Autodesk Inventor part; units mm, degrees
ref_plane "Work Plane2" through (-20, -2, 5) normal (0, 0, 1) x (1, 0, 0)
ref_plane "YZ Plane" through (0, 0, 0) normal (1, 0, 0) x (0, 1, 0)
ref_plane "XZ Plane" through (0, 0, 0) normal (0, 1, 0) x (-1, 0, 0)
sketch "Sketch1" plane through (0, 0, 0) normal (0, 1, 0) x (-1, 0, 0)
  line L0 (0, 0) -> (30, 0)
  line L1 (0, 5) -> (0, 0)
  line L2 (20, 5) -> (30, 0)
  line L3 (30, 12) -> (0, 12)
  line L4 (0, 12) -> (0, 5)
  line L5 (0, 5) -> (0, 7)
  line L6 (18, 7) -> (30, 12)
  line L7 (20, 5) -> (10, 5)
  line L8 (10, 5) -> (10, 7)
  line L9 (18, 7) -> (10, 7)
  line L10 (10, 5) -> (0, 5)
  line L11 (10, 5) -> (10, 0)
  dimension "d13" = 2
  dimension "d15" = 10
extrude "Extrusion2" add sketch "Sketch1" along normal blind 30 contours L1 L10 L11 L0 | L11 L7 L2 L0
ref_plane "Work Plane2" through (-20, -2, 5) normal (0, 0, 1) x (1, 0, 0)
sketch "Sketch2" plane through (-20, -2, 5) normal (0, 0, 1) x (1, 0, 0)
  line L0 (20, 2) -> (20, 17)
  line L1 (20, 2) -> (20, 32)
  line L2 (20, 17) -> (10, 17)
  circle A0 centre (10, 17) radius 5
  circle A1 centre (10, 17) radius 7.5
  line L3 (20, 32) -> (15, 32)
  line L4 (20, 32) -> (-10, 32)
  line L5 (15, 32) -> (15, 27)
  circle A2 centre (15, 27) radius 2.25
  line L6 (20, 17) -> (20, 7)
  line L7 (20, 2) -> (20, 32)
  line L8 (20, 7) -> (15, 7)
  circle A3 centre (15, 7) radius 2.25
  dimension "d20" = 10
  dimension "d21" = 10
  dimension "d22" = 15
  dimension "d30" = 5
  dimension "d31" = 5
  dimension "d32" = 4.5
  dimension "d33" = 10
  dimension "d34" = 5
  dimension "d35" = 4.5
extrude "Extrusion3" cut sketch "Sketch2" against normal blind 3 contours A0
fillet "Fillet3" radius 3 2 edges at (-15, 15, 5) (-15, 15, 2)
extrude "Extrusion4" add sketch "Sketch1" against normal blind 2 contours L11 L7 L2 L0
extrude "Extrusion5" cut sketch "Sketch2" against normal blind 20 contours A2 | A3
properties part number "clip_tip"
For this review, take the finished solid that the model builds, in its own axes (mm). A direction names the side the tool comes from. Coordinates: 2 decimals unless noted, no trailing zeros. Write each loop counter-clockwise with the first axis right and the second up, starting at its lowest first coordinate (ties: lowest second). Pieces come first, ordered by that corner, then holes. Notation, with made-up numbers: (84.5, 53.5) -> (136.5, 53.5) arc R15 cw to (136.5, 81.5) -> close; hole circle Ø5 at (-32.5, 78.5). An arc over 180 degrees is marked (long way). Write each question's results on one line, items separated by ' | '. Start each with the question number.
1) Consider section D-D (z = 4.5). Write out the cut boundary in (x, y), plus the area to 3 significant figures.
2) Consider section A-A (z = 0.9). Write out the cut boundary in (x, y).
3) Consider section C-C (x = -6). Give the number of separate pieces and of enclosed holes in the cut face, plus the area to 3 significant figures.
4) Insertion check: pin 1 (1.5 mm diameter, centred on x = -5, y = 16, fed in from +Z); pin 2 (7 mm diameter, centred on x = -5, y = 5, fed in from -Z); pin 3 (3 mm diameter, centred on x = -6.5, z = 4.5, fed in from -Y); pin 4 (1.5 mm diameter, centred on x = -22, y = 7, fed in from +Z) (3 decimals). Each pin has a flat end and moves straight along its axis. Give the tip position at first contact, or say it passes through.
5) For faces 1 (the face through (-18, -2, 3)), 2 (the face through (-10, -1, 3)), 3 (the face through (-10, 15, 2)), list the 3-axis set-ups (+Z, -Z, +X, -X, +Y, -Y) from which the entire face can be reached by the end or side of a thin tool; tool diameter is ignored.
6) Consider section B-B (y = 25). Write out the cut boundary in (x, z), plus the area to 4 significant figures.
7) Wall thickness on L1, parallel to Y at x = -5, z = 1.45; L2, parallel to Y at x = -3, z = 2.65; L3, parallel to Y at x = -6, z = 4.5: over which ranges is each line inside the solid? List them lowest first. Write a range as [from, to].
8) The part is to be moulded in two halves that separate along X. For faces 4 (the face through (-2.854, 5.676, 2.535)), 5 (the face through (-11, 30, 3)), 6 (the face through (-5.488, 22.804, 2.535)), 7 (the face through (-24.93, 14.224, 2.535)), say which applies: +X half, -X half, draft (parallel to the pull), parting line (faces both ways), or undercut.
Geometry says:
1) outline: (-21, -2) -> (-10, -2) -> (-10, 0) -> (0, 0) -> (0, 30) -> (-21, 30) -> close; hole circle Ø12.68 at (-10, 15); hole circle Ø4.5 at (-5, 5); hole circle Ø4.5 at (-5, 25) | area: 494 mm^2
2) outline: (-28.2, -2) -> (-10, -2) -> (-10, 0) -> (0, 0) -> (0, 30) -> (-28.2, 30) -> close; hole circle Ø4.5 at (-5, 5); hole circle Ø4.5 at (-5, 25)
3) separate pieces: 3 | enclosed holes: 0 | area: 89.1 mm^2
4) pin 1: z = 4.09 | pin 2: z = 0 | pin 3: y = 0 | pin 4: z = 4.375
5) face 1: +Z, -Z, +X, -X, -Y | face 2: +Z, -Z, +X, -Y | face 3: +Z
6) outline: (-30, 0) -> (-7.25, 0) -> (-7.25, 5) -> (-20, 5) -> close; (-2.75, 0) -> (0, 0) -> (0, 5) -> (-2.75, 5) -> close | area: 102.5 mm^2
7) L1: [0, 2.75], [7.25, 22.75], [27.25, 30] | L2: [0, 3.97], [6.03, 23.97], [26.03, 30] | L3: [0, 2.98], [7.02, 10.08], [19.92, 22.98], [27.02, 30]
8) face 4: undercut | face 5: draft | face 6: undercut | face 7: -X half
